```python
from build123d import *

# Parameters (mm, degrees)
F0_R     = 9.525
F1_DEPTH = 25.4
F0_R_2   = 19.05
F2_DEPTH = 50.8
F0_R_3   = 12.7
F3_DEPTH = 25.4


with BuildPart() as f1:
    # F0 (on Top) → F1 (new body)
    with BuildSketch(Plane.XY):
        with BuildLine():
            ThreePointArc((-19.7731447858, -24.8412005603), (-31.75, 0), (-19.7731447858, 24.8412005603))
            Line((-19.7731447858, 24.8412005603), (-53.1594258137, 24.8412005603))
            ThreePointArc((-53.1594258137, 24.8412005603), (-70.9212738909, 17.598203421), (-78.5532782821, 0))
            ThreePointArc((-78.5532782821, 0), (-70.9212738909, -17.598203421), (-53.1594258137, -24.8412005603))
            Line((-53.1594258137, -24.8412005603), (-19.7731447858, -24.8412005603))
        make_face()
        with Locations((-50.8, 0)):
            Circle(F0_R, mode=Mode.SUBTRACT)
    extrude(amount=F1_DEPTH)

    # F0 (on Top) → F2 (join)
    with BuildSketch(Plane.XY):
        with BuildLine():
            ThreePointArc((-19.7731447858, -24.8412005603), (0, -31.75), (19.7731447858, -24.8412005603))
            Line((19.7731447858, -24.8412005603), (-19.7731447858, -24.8412005603))
        make_face()
        with BuildLine():
            Line((-19.7731447858, 24.8412005603), (19.7731447858, 24.8412005603))
            ThreePointArc((19.7731447858, 24.8412005603), (0, 31.75), (-19.7731447858, 24.8412005603))
        make_face()
        with BuildLine():
            ThreePointArc((19.7731447858, -24.8412005603), (28.5994741818, -13.7888569695), (31.75, 0))
            ThreePointArc((31.75, 0), (28.5994741818, 13.7888569695), (19.7731447858, 24.8412005603))
            Line((19.7731447858, 24.8412005603), (-19.7731447858, 24.8412005603))
            ThreePointArc((-19.7731447858, 24.8412005603), (-31.75, 0), (-19.7731447858, -24.8412005603))
            Line((-19.7731447858, -24.8412005603), (19.7731447858, -24.8412005603))
        make_face()
        Circle(F0_R_2, mode=Mode.SUBTRACT)
    extrude(amount=F2_DEPTH)

    # F0 (on Top) → F3 (join)
    with BuildSketch(Plane.XY):
        with BuildLine():
            ThreePointArc((19.7731447858, 24.8412005603), (28.5994741818, 13.7888569695), (31.75, 0))
            ThreePointArc((31.75, 0), (28.5994741818, -13.7888569695), (19.7731447858, -24.8412005603))
            Line((19.7731447858, -24.8412005603), (70.5508692495, -24.8412005603))
            ThreePointArc((70.5508692495, -24.8412005603), (88.3127173267, -17.598203421), (95.9447217179, 0))
            ThreePointArc((95.9447217179, 0), (88.3127173267, 17.598203421), (70.5508692495, 24.8412005603))
            Line((70.5508692495, 24.8412005603), (19.7731447858, 24.8412005603))
        make_face()
        with BuildLine():
            ThreePointArc((39.3356828899, -0.5587994397), (41.3437381638, 3.6329638912), (45.6692023039, 5.3340005688))
            Line((45.6692023039, 5.3340005688), (73.6092023039, 5.3340005688))
            ThreePointArc((73.6092023039, 5.3340005688), (77.934666444, 3.6329638912), (79.9427217179, -0.5587994397))
            ThreePointArc((79.9427217179, -0.5587994397), (77.934666444, -4.7505627706), (73.6092023039, -6.4515994482))
            Line((73.6092023039, -6.4515994482), (45.6692023039, -6.4515994482))
            ThreePointArc((45.6692023039, -6.4515994482), (41.3437381638, -4.7505627706), (39.3356828899, -0.5587994397))
        make_face(mode=Mode.SUBTRACT)
        Circle(F0_R_2)
        Circle(F0_R_3, mode=Mode.SUBTRACT)
    extrude(amount=F3_DEPTH)


solid = f1.part
```
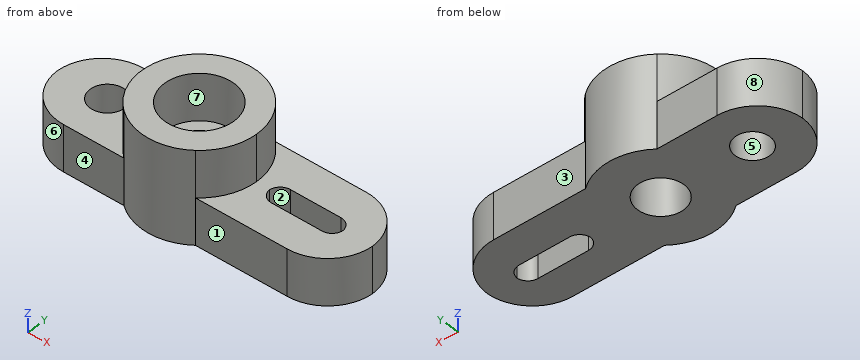
Here's how the part is built. I have some questions about the finished solid (model axes, mm). Face numbers are marked on the shaded views. A direction names the side the tool comes from. Round coordinates to 2 decimals unless told otherwise and drop trailing zeros. Loops run counter-clockwise (first coordinate to the right, second up) from the corner with the lowest first, then second, coordinate; pieces in that order, holes last. Notation, with made-up numbers: (58.25, 58) -> (111.25, 58) arc R29 cw to (111.25, 78) -> close; hole circle Ø5 at (27.25, 67.5). An arc over 180 degrees is marked (long way). Answer as CSV lines item,"result". Start each with the question number.
1. I need wall thicknesses on probe 1 along Y at (x, z) = (0, 36); probe 2 along Y at (x, z) = (0, 5.5); probe 3 along X at (y, z) = (2.5, 23.5). Which ranges of each line are inside material? Lowest first, please. Write a range as from..to.
2. Imagine slicing it at A-A on x = 0. Write out the boundary of the cut face in (y, z).
3. For the marked faces 1, 2, 3 and 4, which set-ups out of +Z, -Z, +X, -X, +Y, -Y let a thin tool reach every point of the face, with its end or its side?
4. Imagine slicing it at B-B on z = 16. Write out the boundary of the cut face in (x, y) (3 decimals), plus the area to 3 significant figures.
5. I'm going to push flat-ended pins straight in: P1, Ø12, axis at x = 44.5, y = 4, coming from the +Z side; P2, Ø15, axis at x = 0, y = 0, coming from the -Z side; P3, Ø1.5, axis at y = 19, z = 24.5, coming from the -X side; P4, Ø20.5, axis at x = -44.5, z = 18, coming from the +Y side. Where does each tip first touch, or does it pass through?
6. If we mould it in two halves opening along Y, with no side actions, what happens to the marked faces 5, 6, 7 and 8? For each: pulls with the +Y half, pulls with the -Y half, needs draft (parallel to the pull), parting line crosses it, or undercut.
7. Imagine slicing it at C-C on x = -50.8. Write out the boundary of the cut face in (y, z) (3 decimals), plus the area to 3 significant figures.
8. Imagine slicing it at D-D on z = 37. Write out the boundary of the cut face in (x, y), plus the area to 3 significant figures.
Solution:
1,probe 1,"-31.75..-19.05, 19.05..31.75"
1,probe 2,"-31.75..-12.7, 12.7..31.75"
1,probe 3,"-78.37..-59.99, -41.61..-12.45, 12.45..40.38, 78.9..95.77"
2,outline,"(-31.75, 0) -> (-12.7, 0) -> (-12.7, 25.4) -> (-19.05, 25.4) -> (-19.05, 50.8) -> (-31.75, 50.8) -> close; (12.7, 0) -> (31.75, 0) -> (31.75, 50.8) -> (19.05, 50.8) -> (19.05, 25.4) -> (12.7, 25.4) -> close"
3,face 1,"+Z, -Z, +X, -Y"
3,face 2,"+Z, -Z"
3,face 3,"+Z, -Z, +X, +Y"
3,face 4,"+Z, -Z, -X, -Y"
4,outline,"(-78.553, 0) arc R25.4 ccw to (-53.159, -24.841) -> (-19.773, -24.841) arc R31.75 ccw to (19.773, -24.841) -> (70.551, -24.841) arc R25.4 ccw to (95.945, 0) arc R25.4 ccw to (70.551, 24.841) -> (19.773, 24.841) arc R31.75 ccw to (-19.773, 24.841) -> (-53.159, 24.841) arc R25.4 ccw to start; hole circle Ø19.05 at (-50.8, 0); hole circle Ø25.4 at (0, 0); hole (39.336, -0.559) arc R6.35 ccw to (45.669, -6.452) -> (73.609, -6.452) arc R6.35 ccw to (79.943, -0.559) arc R6.35 ccw to (73.609, 5.334) -> (45.669, 5.334) arc R6.35 ccw to start"
4,area,"7,250 mm²"
5,P1,"z = 25.4"
5,P2,"through"
5,P3,"x = -70.23"
5,P4,"y = 24.84"
6,face 5,"undercut"
6,face 6,"pulls with the -Y half"
6,face 7,"undercut"
6,face 8,"pulls with the +Y half"
7,outline,"(-24.841, 0) -> (-9.525, 0) -> (-9.525, 25.4) -> (-24.841, 25.4) -> close; (9.525, 0) -> (24.841, 0) -> (24.841, 25.4) -> (9.525, 25.4) -> close"
7,area,"778 mm²"
8,outline,"circle Ø63.5 at (0, 0); hole circle Ø38.1 at (0, 0)"
8,area,"2,030 mm²"
